```python
from build123d import *

# Parameters (mm, degrees)
EXTRUDE_1_DEPTH          = 10
CUT_EXTRUDE_1_REACH      = 82.25
SKETCH_3_W               = 40
SKETCH_3_H               = 10
CUT_EXTRUDE_2_REACH      = 82.92
SKETCH_4_R               = 2.5
SKETCH_5_R               = 27.5
EXTRUDE_2_DEPTH          = 5
CUT_EXTRUDE_3_REACH      = 87.09
SKETCH_6_R               = 1.6
PATTERN_CIRCULAR_1_COUNT = 6
SKETCH_7_R               = 12.5
EXTRUDE_3_DEPTH          = 10
SKETCH_8_R               = 4
EXTRUDE_4_DEPTH          = 2
SKETCH_9_R               = 2.5
EXTRUDE_5_DEPTH          = 5


with BuildPart() as part:
    # 草图2 → 凸台-拉伸1 (new, symmetric)
    with BuildSketch(Plane(origin=(0, 0, 0), x_dir=(1, 0, 0), z_dir=(0, 1, 0))):
        with BuildLine():
            Line((0, 8), (70, 8))
            ThreePointArc((70, 8), (78, 0), (70, -8))
            Line((70, -8), (0, -8))
            ThreePointArc((0, -8), (-8, 0), (0, 8))
        make_face()
    extrude(amount=EXTRUDE_1_DEPTH, both=True)

    # 草图3 → 切除-拉伸1 (cut, up to next)
    with BuildSketch(Plane.XY.offset(8), mode=Mode.PRIVATE) as cut_extrude_1_sk1:
        with Locations((58, 0)):
            Rectangle(SKETCH_3_W, SKETCH_3_H)
    cut_extrude_1_tool1 = extrude(cut_extrude_1_sk1.sketch, amount=-CUT_EXTRUDE_1_REACH, mode=Mode.PRIVATE) & part.part
    add(cut_extrude_1_tool1.solids().sort_by_distance((58, 0, 8))[0], mode=Mode.SUBTRACT)

    # 切除-拉伸2: up to this face of the body (flat: up to its plane)
    cut_extrude_2_end = Plane(part.part.faces().sort_by_distance((35, -10, 0))[0])
    # 草图4 → 切除-拉伸2 (cut, up to the picked face)
    with BuildSketch(Plane(origin=(0, 10, 0), x_dir=(1, 0, 0), z_dir=(0, 1, 0)), mode=Mode.PRIVATE) as cut_extrude_2_sk1:
        with Locations(Location((70, 0, 0), (0, 0, 270))):
            Circle(SKETCH_4_R)
    cut_extrude_2_tool1 = split(extrude(cut_extrude_2_sk1.sketch, amount=-CUT_EXTRUDE_2_REACH, mode=Mode.PRIVATE), bisect_by=cut_extrude_2_end, keep=Keep.BOTH, mode=Mode.PRIVATE)
    add(cut_extrude_2_tool1.solids().sort_by(Axis((70, 10, 0), (0, -1, 0)))[0], mode=Mode.SUBTRACT)

    # 草图5 → 凸台-拉伸2 (add)
    with BuildSketch(Plane.XZ.offset(10)):
        with Locations(Location((0, 0, 0), (0, 0, 16.912389803))):
            Circle(SKETCH_5_R)
    extrude(amount=EXTRUDE_2_DEPTH)

    # 草图6 → 切除-拉伸3 (cut, up to next)
    with BuildSketch(Plane(origin=(0, -10, 0), x_dir=(1, 0, 0), z_dir=(0, 1, 0)), mode=Mode.PRIVATE) as cut_extrude_3_sk1:
        with Locations(Location((0, 24, 0), (0, 0, 270))):
            Circle(SKETCH_6_R)
    cut_extrude_3_tool1 = extrude(cut_extrude_3_sk1.sketch, amount=-CUT_EXTRUDE_3_REACH, mode=Mode.PRIVATE) & part.part
    cut_extrude_3 = cut_extrude_3_tool1.solids().sort_by_distance((0, -10, -24))[0]
    add(cut_extrude_3, mode=Mode.SUBTRACT)

    # 阵列(圆周)1: 切除-拉伸3 ×6 about axis
    pattern_circular_1_axis = Axis((0, 0, 0), (0, 1, 0))
    for i in range(1, PATTERN_CIRCULAR_1_COUNT):
        add(cut_extrude_3.rotate(pattern_circular_1_axis, i * 360 / PATTERN_CIRCULAR_1_COUNT), mode=Mode.SUBTRACT)

    # 草图7 → 凸台-拉伸3 (add)
    with BuildSketch(Plane(origin=(0, -10, 0), x_dir=(1, 0, 0), z_dir=(0, 1, 0))):
        Circle(SKETCH_7_R)
    extrude(amount=EXTRUDE_3_DEPTH)

    # 草图8 → 凸台-拉伸4 (add)
    with BuildSketch(Plane(origin=(0, 10, 0), x_dir=(1, 0, 0), z_dir=(0, 1, 0))):
        with Locations(Location((0, 0, 0), (0, 0, 270))):
            Circle(SKETCH_8_R)
    extrude(amount=EXTRUDE_4_DEPTH)

    # 草图9 → 凸台-拉伸5 (add)
    with BuildSketch(Plane(origin=(0, 12, 0), x_dir=(1, 0, 0), z_dir=(0, 1, 0))):
        with Locations(Location((0, 0, 0), (0, 0, 270))):
            Circle(SKETCH_9_R)
    extrude(amount=EXTRUDE_5_DEPTH)


solid = part.part
```
Build history of the part. All positions in model axes, mm. A direction names the side the tool comes from. Round coordinates to 2 decimals unless told otherwise and drop trailing zeros. Write each loop counter-clockwise with the first axis right and the second up, starting at its lowest first coordinate (ties: lowest second). Pieces come first, ordered by that corner, then holes.
1) Band-saw the part on C-C, the plane z = -24. List the corners of the cut face in (x, y).
2) Drill centre lines: probe 1 along X at (y, z) = (-13, -12); probe 2 along X at (y, z) = (6, 0); probe 3 along Y at (x, z) = (69, -3). Where is each one in solid material? Low to high.
3) Band-saw the part on A-A, the plane z = 0. Give the number of separate pieces and of enclosed holes in the cut face, and give its area (3 significant figures).
4) Mould opens along X. For faces 1 (the flat face through (58, 5, 0)), 2 (the cylindrical face through (-12.493, -5.07, -0.428)), 3 (the cylindrical face through (19.703, -12.465, -10.821)) say: +X half, -X half, draft (parallel to the pull), parting line (faces both ways), or undercut.
5) Band-saw the part on D-D, the plane x = 13.5. List the corners of the cut face in (y, z), and give its area (3 significant figures).
6) Pin check, flat tips, straight feed: pin 1 (16 mm diameter, centred on x = 47, y = -1.5, fed in from -Z); pin 2 (6 mm diameter, centred on x = 70, z = 0, fed in from -Y); pin 3 (4 mm diameter, centred on y = -1.5, z = -6, fed in from +X); pin 4 (2 mm diameter, centred on y = 4.5, z = -1, fed in from +X). Stop position of each tip, or through.
7) 3-axis set-ups, long thin cutter, end or side, ignore diameter. For faces 4 (the flat face through (58, -5, 0)), 5 (the flat face through (-9, 0, 0)), 6 (the flat face through (27, 0, -8)): which of +Z, -Z, +X, -X, +Y, -Y reach the whole face in a straight line?
8) Band-saw the part on B-B, the plane y = -8. List the corners of the cut face in (x, z), and give its area (3 significant figures).
Ans:
1. outline: (-13.43, -15) - (-1.6, -15) - (-1.6, -10) - (-13.43, -10) - close; (1.6, -15) - (13.43, -15) - (13.43, -10) - (1.6, -10) - close
2. probe 1: x = -24.74 to -22.38, -19.18 to 19.18, 22.38 to 24.74
2. probe 2: x = -8 to 67.5, 72.5 to 78
2. probe 3: y = -10 to -5, 5 to 10
3. separate pieces: 3
3. enclosed holes: 0
3. area: 1,630 mm2
4. face 1: draft
4. face 2: parting line
4. face 3: undercut
5. outline: (-15, -23.96) - (-10, -23.96) - (-10, -8) - (10, -8) - (10, 8) - (-10, 8) - (-10, 23.96) - (-15, 23.96) - close
5. area: 560 mm2
6. pin 1: stops at z = -8
6. pin 2: stops at y = -10
6. pin 3: stops at x = 38
6. pin 4: stops at x = 78
7. face 4: +Z, -Z, +X
7. face 5: -X, +Y
7. face 6: -Z, +X, +Y
8. outline: (9.6, -8) - (70, -8) arc R8 ccw to (70, 8) - (9.6, 8) arc R12.5 ccw (long way) to start; hole circle Ø5 at (70, 0)
8. area: 1,510 mm2
